Job drawing, mm, ordinate dimensions from the low corner. One solid piece. A direction names the side the tool comes from. Coordinates: 2 decimals unless noted, no trailing zeros. Loops run counter-clockwise (first coordinate to the right, second up) from the corner with the lowest first, then second, coordinate; pieces in that order, holes last. Notation, with made-up numbers: (-33.5, 33.25) - (25.5, 33.25) arc R28 cw to (25.5, 62.25) - close; hole circle Ø9 at (19.5, 6). An arc over 180 degrees is marked (long way). Use a Markdown table: item, result. Add a question column.
1) Tool access for the marked faces 1 and 2: list every direction of +Z, -Z, +X, -X, +Y, -Y with a clear straight run to the whole face (end or side of a thin tool).
2) Band-saw the part on B-B (y = 14.25). Give the cut face in (x, z), plus the area to 3 significant figures.
3) Band-saw the part on C-C (y = 2). Give the cut face in (x, z).
4) Drop flat-ended pins along their axis: P1, Ø5.5, axis at x = 25.5, y = 7.5, coming from the +Z side; P2, Ø2, axis at y = 10, z = 11.5, coming from the -X side; P3, Ø3, axis at y = 12, z = 15.5, coming from the +X side. Give the stop position or say it passes through.
5) Band-saw the part on A-A (x = 15). Give the cut face in (y, z), plus the area to 3 significant figures.
6) Probe probe 1 along X at (y, z) = (1.25, 15); probe 2 along X at (y, z) = (7, 13.5); probe 3 along Y at (x, z) = (27.3, 15). List the from-to ranges inside material, lowest first. Write a range as [from, to].
7) Band-saw the part on D-D (z = 12.25). Give the cut face in (x, y).
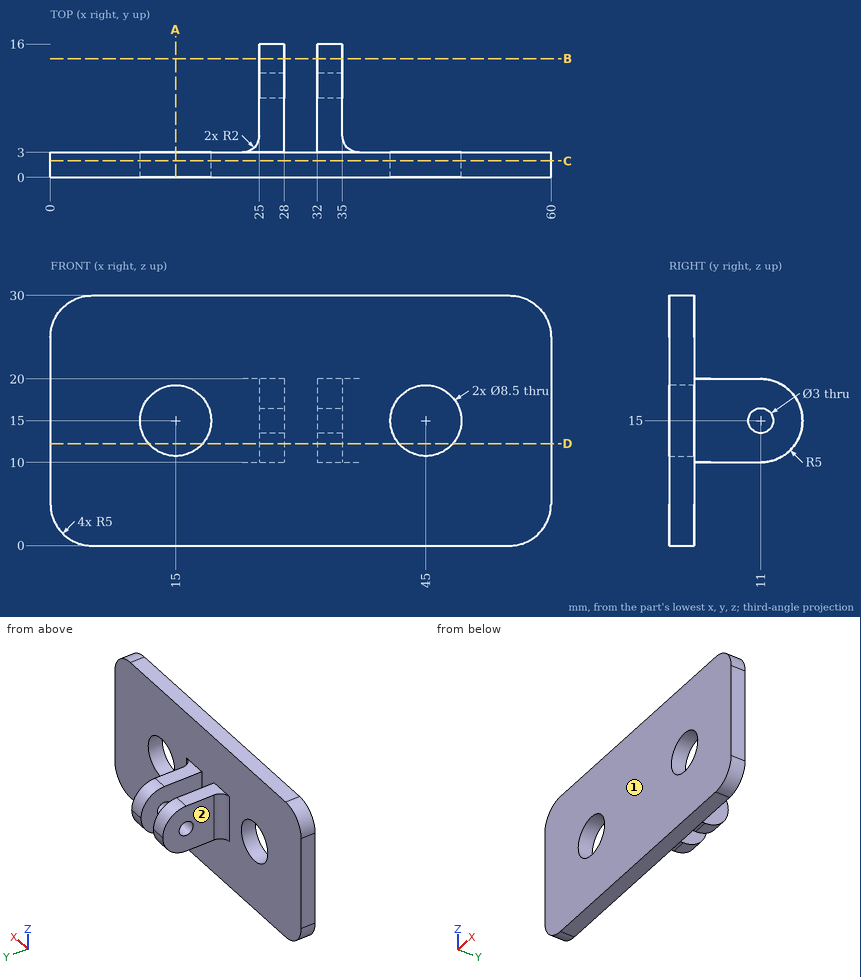
Answer block:
| question | item | result |
|---|---|---|
| 1 | face 1 | +Z, -Z, +X, -X, -Y |
| 1 | face 2 | +Z, -Z, -X, +Y |
| 2 | outline | (25, 11.2) - (28, 11.2) - (28, 18.8) - (25, 18.8) - close; (32, 11.2) - (35, 11.2) - (35, 18.8) - (32, 18.8) - close |
| 2 | area | 45.6 mm2 |
| 3 | outline | (0, 5) arc R5 ccw to (5, 0) - (55, 0) arc R5 ccw to (60, 5) - (60, 25) arc R5 ccw to (55, 30) - (5, 30) arc R5 ccw to (0, 25) - close; hole circle Ø8.5 at (15, 15); hole circle Ø8.5 at (45, 15) |
| 4 | P1 | z = 20 |
| 4 | P2 | x = 25 |
| 4 | P3 | x = 35 |
| 5 | outline | (0, 0) - (3, 0) - (3, 10.75) - (0, 10.75) - close; (0, 19.25) - (3, 19.25) - (3, 30) - (0, 30) - close |
| 5 | area | 64.5 mm2 |
| 6 | probe 1 | [0, 10.75], [19.25, 40.75], [49.25, 60] |
| 6 | probe 2 | [25, 28], [32, 35] |
| 6 | probe 3 | [0, 9.5], [12.5, 16] |
| 7 | outline | (0, 0) - (11.76, 0) - (11.76, 3) - (0, 3) - close; (18.24, 0) - (41.76, 0) - (41.76, 3) - (37, 3) arc R2 cw to (35, 5) - (35, 15.18) - (32, 15.18) - (32, 3) - (28, 3) - (28, 15.18) - (25, 15.18) - (25, 5) arc R2 cw to (23, 3) - (18.24, 3) - close; (48.24, 0) - (60, 0) - (60, 3) - (48.24, 3) - close |
